Job drawing, mm, ordinate dimensions from the low corner. One solid piece. A direction names the side the tool comes from. Coordinates: 2 decimals unless noted, no trailing zeros. Write each loop counter-clockwise with the first axis right and the second up, starting at its lowest first coordinate (ties: lowest second). Pieces come first, ordered by that corner, then holes. Notation, with made-up numbers: (-36.75, -8.75) -> (-13.75, -8.75) arc R11 cw to (-13.75, 3.25) -> close; hole circle Ø1 at (14.5, -9). An arc over 180 degrees is marked (long way). Answer as a JSON object with one key per item and string values. Group by question number.
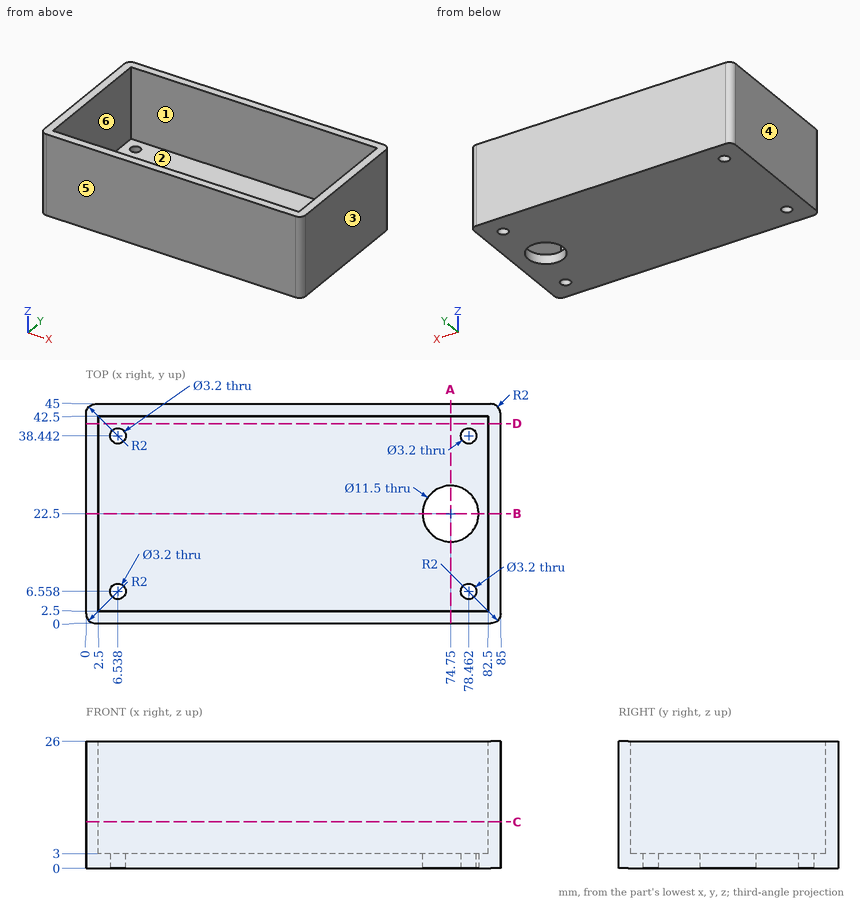
(1) Cut at D-D on y = 41. List the corners of the cut face in (x, z), plus the area to 3 significant figures.
(2) Pin check, flat tips, straight feed: pin 1 (8 mm diameter, centred on x = 47, y = 10, fed in from +Z); pin 2 (4 mm diameter, centred on x = 78.462, y = 6.558, fed in from -Z). Stop position of each tip, or through.
(3) Cut at C-C on z = 9.5. List the corners of the cut face in (x, y), plus the area to 3 significant figures.
(4) Cut at B-B on y = 22.5. List the corners of the cut face in (x, z), plus the area to 4 significant figures.
(5) 3-axis set-ups, long thin cutter, end or side, ignore diameter. For the marked faces 5 and 6: which of +Z, -Z, +X, -X, +Y, -Y reach the whole face in a straight line?
(6) Cut at A-A on x = 74.75. List the corners of the cut face in (y, z), plus the area to 4 significant figures.
(7) Wall check: probe 1 along Y at (x, z) = (16.5, 15); probe 2 along X at (y, z) = (33, 18); probe 3 along Z at (x, y) = (72.5, 28.5). Give the ranges that are in metal, low to high.
(8) Pull direction X, two halves, no side cores. Call the marked faces 1, 2, 3 and 4: released by +X, released by -X, zero draft, split by the parting line, or undercut.
Results found:
{
 "1": {"outline": "(0, 0) -> (85, 0) -> (85, 26) -> (82.5, 26) -> (82.5, 3) -> (2.5, 3) -> (2.5, 26) -> (0, 26) -> close", "area": "370 mm²"},
 "2": {"pin 1": "stops at z = 3", "pin 2": "stops at z = 0"},
 "3": {"outline": "(0, 2) arc R2 ccw to (2, 0) -> (83, 0) arc R2 ccw to (85, 2) -> (85, 43) arc R2 ccw to (83, 45) -> (2, 45) arc R2 ccw to (0, 43) -> close; hole (2.5, 2.5) -> (82.5, 2.5) -> (82.5, 42.5) -> (2.5, 42.5) -> close", "area": "622 mm²"},
 "4": {"outline": "(0, 0) -> (69, 0) -> (69, 3) -> (2.5, 3) -> (2.5, 26) -> (0, 26) -> close; (80.5, 0) -> (85, 0) -> (85, 26) -> (82.5, 26) -> (82.5, 3) -> (80.5, 3) -> close", "area": "335.5 mm²"},
 "5": {"face 5": "+Z, -Z, +X, -X, -Y", "face 6": "+Z"},
 "6": {"outline": "(0, 0) -> (16.75, 0) -> (16.75, 3) -> (2.5, 3) -> (2.5, 26) -> (0, 26) -> close; (28.25, 0) -> (45, 0) -> (45, 26) -> (42.5, 26) -> (42.5, 3) -> (28.25, 3) -> close", "area": "215.5 mm²"},
 "7": {"probe 1": "y = 0 to 2.5, 42.5 to 45", "probe 2": "x = 0 to 2.5, 82.5 to 85", "probe 3": "z = 0 to 3"},
 "8": {"face 1": "undercut", "face 2": "undercut", "face 3": "released by +X", "face 4": "released by -X"}
}
